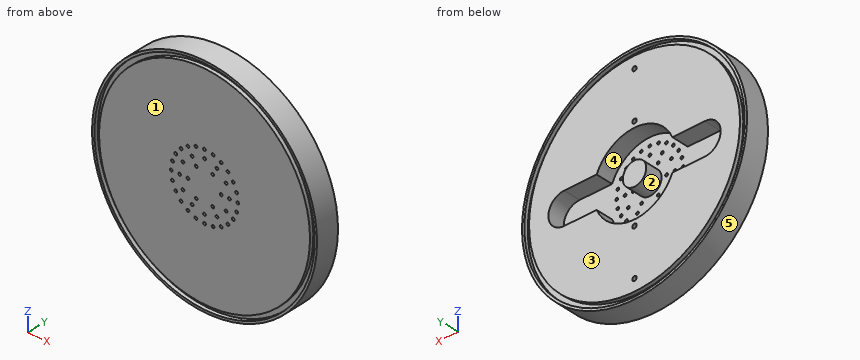
```python
from build123d import *

# Parameters (mm, degrees)
SKETCH1_R                       = 60.96
BILLET_DEPTH                    = 12.7
SKETCH4_R                       = 0.7493
FIRST_KEROSENE_OUTLET_DEPTH     = 88.140881336
SKETCH15_R                      = 59.69
SKETCH15_R_2                    = 57.15
CHAMBER_O_RING_DEPTH            = 2.032
TOP_START                       = -2.032
SKETCH16_R                      = 59.69
SKETCH16_R_2                    = 57.15
TOP_O_RING_DEPTH                = 2.032
PRIMARY_HOLES_COUNT             = 6
SECOND_START                    = -12.7
SECOND_RING_OUTLINE_R           = 0.7493
SECOND_RING_DEPTH               = 12.7
THIRD_START                     = -12.7
THIRD_RING_OUTLINE_R            = 0.7493
THIRD_RING_DEPTH                = 12.7
KEROSENE_WELL_DEPTH             = 9.3218
SKETCH17_R                      = 6.35
BOSS_EXTRUDE1_DEPTH             = 2.54
BOSS_EXTRUDE1_DIRECTION_2_REACH = 89.141
SKETCH19_R                      = 6.35
LOX_TOWER_DEPTH                 = 2.54
SKETCH20_R                      = 1.190625
DOWELS_DEPTH                    = 3.175


# Read off the part's stored shape, not the designer's step: Second ring, Third Ring
with BuildPart() as part:
    # Sketch1 → Billet (new body)
    with BuildSketch(Plane(origin=(0, 0, 0), x_dir=(1, 0, 0), z_dir=(0, 1, 0))):
        with Locations(Location((0, 0, 0), (0, 0, 270))):
            Circle(SKETCH1_R)
    extrude(amount=-BILLET_DEPTH)

    # Sketch4 → First Kerosene Outlet (cut, symmetric)
    with BuildSketch(Plane(origin=(0, -12.7, 0), x_dir=(1, 0, 0), z_dir=(0, 1, 0))):
        with Locations(Location((8.9916, 0, 0), (0, 0, 270))):
            Circle(SKETCH4_R)
        with Locations(Location((13.4874, 0, 0), (0, 0, 270))):
            Circle(SKETCH4_R)
        with Locations(Location((17.9832, 0, 0), (0, 0, 270))):
            Circle(SKETCH4_R)
    first_kerosene_outlet = extrude(amount=FIRST_KEROSENE_OUTLET_DEPTH, both=True, mode=Mode.SUBTRACT)

    # Sketch15 → Chamber O Ring (cut)
    with BuildSketch(Plane(origin=(0, -12.7, 0), x_dir=(1, 0, 0), z_dir=(0, 1, 0))):
        with Locations(Location((0, 0, 0), (0, 0, 270))):
            Circle(SKETCH15_R)
        with Locations(Location((0, 0, 0), (0, 0, 270))):
            Circle(SKETCH15_R_2, mode=Mode.SUBTRACT)
    extrude(amount=CHAMBER_O_RING_DEPTH, mode=Mode.SUBTRACT)

    # Sketch16 → Top O ring (cut)
    with BuildSketch(Plane(origin=(0, 0, 0), x_dir=(1, 0, 0), z_dir=(0, 1, 0)).offset(TOP_START)):
        with Locations(Location((0, 0, 0), (0, 0, 270))):
            Circle(SKETCH16_R)
        with Locations(Location((0, 0, 0), (0, 0, 270))):
            Circle(SKETCH16_R_2, mode=Mode.SUBTRACT)
    extrude(amount=TOP_O_RING_DEPTH, mode=Mode.SUBTRACT)

    # Primary Holes: First Kerosene Outlet ×6 about axis
    primary_holes_axis = Axis((0, 0, 0), (0, 1, 0))
    for i in range(1, PRIMARY_HOLES_COUNT):
        add(first_kerosene_outlet.rotate(primary_holes_axis, i * 360 / PRIMARY_HOLES_COUNT), mode=Mode.SUBTRACT)

    # Second ring outline → Second ring (cut)
    with BuildSketch(Plane(origin=(0, 0, 0), x_dir=(1, 0, 0), z_dir=(0, 1, 0)).offset(SECOND_START)):
        with Locations((11.680431031, 6.7437)):
            Circle(SECOND_RING_OUTLINE_R)
        with Locations((0, 13.4874)):
            Circle(SECOND_RING_OUTLINE_R)
        with Locations((-11.680431031, 6.7437)):
            Circle(SECOND_RING_OUTLINE_R)
        with Locations((-11.680431031, -6.7437)):
            Circle(SECOND_RING_OUTLINE_R)
        with Locations((0, -13.4874)):
            Circle(SECOND_RING_OUTLINE_R)
        with Locations((11.680431031, -6.7437)):
            Circle(SECOND_RING_OUTLINE_R)
    extrude(amount=SECOND_RING_DEPTH, mode=Mode.SUBTRACT)

    # Third Ring outline → Third Ring (cut)
    with BuildSketch(Plane(origin=(0, 0, 0), x_dir=(1, 0, 0), z_dir=(0, 1, 0)).offset(THIRD_START)):
        with Locations((17.370437319, 4.654394652)):
            Circle(THIRD_RING_OUTLINE_R)
        with Locations((15.573908041, 8.9916)):
            Circle(THIRD_RING_OUTLINE_R)
        with Locations((12.716042667, 12.716042667)):
            Circle(THIRD_RING_OUTLINE_R)
        with Locations((4.654394652, 17.370437319)):
            Circle(THIRD_RING_OUTLINE_R)
        with Locations((0, 17.9832)):
            Circle(THIRD_RING_OUTLINE_R)
        with Locations((-4.654394652, 17.370437319)):
            Circle(THIRD_RING_OUTLINE_R)
        with Locations((-12.716042667, 12.716042667)):
            Circle(THIRD_RING_OUTLINE_R)
        with Locations((-15.573908041, 8.9916)):
            Circle(THIRD_RING_OUTLINE_R)
        with Locations((-17.370437319, 4.654394652)):
            Circle(THIRD_RING_OUTLINE_R)
        with Locations((-17.370437319, -4.654394652)):
            Circle(THIRD_RING_OUTLINE_R)
        with Locations((-15.573908041, -8.9916)):
            Circle(THIRD_RING_OUTLINE_R)
        with Locations((-12.716042667, -12.716042667)):
            Circle(THIRD_RING_OUTLINE_R)
        with Locations((-4.654394652, -17.370437319)):
            Circle(THIRD_RING_OUTLINE_R)
        with Locations((0, -17.9832)):
            Circle(THIRD_RING_OUTLINE_R)
        with Locations((4.654394652, -17.370437319)):
            Circle(THIRD_RING_OUTLINE_R)
        with Locations((12.716042667, -12.716042667)):
            Circle(THIRD_RING_OUTLINE_R)
        with Locations((15.573908041, -8.9916)):
            Circle(THIRD_RING_OUTLINE_R)
        with Locations((17.370437319, -4.654394652)):
            Circle(THIRD_RING_OUTLINE_R)
    extrude(amount=THIRD_RING_DEPTH, mode=Mode.SUBTRACT)

    # Sketch18 → Kerosene Well (cut)
    with BuildSketch(Plane(origin=(0, 0, 0), x_dir=(1, 0, 0), z_dir=(0, 1, 0))):
        with BuildLine():
            Line((-38.1, 8.57504), (-20.504129194, 8.57504))
            ThreePointArc((-20.504129194, 8.57504), (0, 22.225), (20.504129194, 8.57504))
            Line((20.504129194, 8.57504), (38.1, 8.57504))
            ThreePointArc((38.1, 8.57504), (46.67504, 0), (38.1, -8.57504))
            Line((38.1, -8.57504), (20.504129194, -8.57504))
            ThreePointArc((20.504129194, -8.57504), (0, -22.225), (-20.504129194, -8.57504))
            Line((-20.504129194, -8.57504), (-38.1, -8.57504))
            ThreePointArc((-38.1, -8.57504), (-46.67504, 0), (-38.1, 8.57504))
        make_face()
    extrude(amount=-KEROSENE_WELL_DEPTH, mode=Mode.SUBTRACT)

    # Sketch17 → Boss-Extrude1 (add)
    with BuildSketch(Plane(origin=(0, 0, 0), x_dir=(1, 0, 0), z_dir=(0, 1, 0))):
        with Locations(Location((0, 0, 0), (0, 0, 270))):
            Circle(SKETCH17_R)
    extrude(amount=BOSS_EXTRUDE1_DEPTH)

    # Sketch17 → Boss-Extrude1 direction 2 (add, up to next)
    with BuildSketch(Plane(origin=(0, 0, 0), x_dir=(1, 0, 0), z_dir=(0, 1, 0)), mode=Mode.PRIVATE) as boss_extrude1_direction_2_sk1:
        with Locations(Location((0, 0, 0), (0, 0, 270))):
            Circle(SKETCH17_R)
    boss_extrude1_direction_2_tool1 = extrude(boss_extrude1_direction_2_sk1.sketch, amount=-BOSS_EXTRUDE1_DIRECTION_2_REACH, mode=Mode.PRIVATE) - part.part
    add(boss_extrude1_direction_2_tool1.solids().sort_by_distance((0, 0, 0))[0])

    # Sketch19 → Lox Tower (cut)
    with BuildSketch(Plane(origin=(0, 2.54, 0), x_dir=(1, 0, 0), z_dir=(0, 1, 0))):
        with Locations(Location((0, 0, 0), (0, 0, 270))):
            Circle(SKETCH19_R)
    extrude(amount=-LOX_TOWER_DEPTH, mode=Mode.SUBTRACT)

    # Sketch20 → Dowels (cut)
    with BuildSketch(Plane(origin=(0, 0, 0), x_dir=(1, 0, 0), z_dir=(0, 1, 0))):
        with Locations(Location((0, 25.4, 0), (0, 0, 270))):
            Circle(SKETCH20_R)
        with Locations(Location((0, -25.4, 0), (0, 0, 90))):
            Circle(SKETCH20_R)
        with Locations(Location((0, 50.8, 0), (0, 0, 270))):
            Circle(SKETCH20_R)
        with Locations(Location((0, -50.8, 0), (0, 0, 90))):
            Circle(SKETCH20_R)
    extrude(amount=-DOWELS_DEPTH, mode=Mode.SUBTRACT)


solid = part.part
```
Can you work these out from the model? Positions are in its coordinate system, mm. Face numbers are marked on the shaded views. A direction names the side the tool comes from. Coordinates: 2 decimals unless noted, no trailing zeros. Loops run counter-clockwise (first coordinate to the right, second up) from the corner with the lowest first, then second, coordinate; pieces in that order, holes last.
1) For pin 1 (1.2 mm diameter, centred on x = 6.74, z = 11.68, fed in from -Y); pin 2 (4 mm diameter, centred on x = 43, y = -7, fed in from +Z); pin 3 (4 mm diameter, centred on y = -4, z = 17.5, fed in from +X); pin 4 (2.5 mm diameter, centred on x = 17.37, z = 4.65, fed in from +Y), each with a flat end and sliding along its axis, tell me the tip position at first contact or that it passes through.
2) Imagine slicing it at B-B on z = -36. List the corners of the cut face in (x, y) for me.
3) Imagine slicing it at A-A on y = -7.5. List the corners of the cut face in (x, z) for me (3 decimals), plus the area to 3 significant figures.
4) Thinking about a two-plate mould opening in X: for the marked faces 3, 4 and 5, which applies, pulls with the +X half, pulls with the -X half, needs draft (parallel to the pull), parting line crosses it, or undercut?
5) Which directions (+Z, -Z, +X, -X, +Y, -Y) give clear straight access to the entire face, cutting with the end or side of a thin tool? Please do the marked faces 1 and 2.
6) I need wall thicknesses on probe 1 along X at (y, z) = (-1.25, -4.5); probe 2 along X at (y, z) = (-10.75, 31); probe 3 along X at (y, z) = (-0.5, 15.5). Which ranges of each line are inside material? Lowest first, please.
7) Imagine slicing it at C-C on x = 26. List the corners of the cut face in (y, z) for me, plus the area to 3 significant figures.
Completed:
1. pin 1: passes through
1. pin 2: stops at z = 45.11
1. pin 3: stops at x = 58.96
1. pin 4: stops at y = -9.32
2. outline: (-49.19, -12.7) - (-47.61, -12.7) - (-47.61, -10.67) - (-44.39, -10.67) - (-44.39, -12.7) - (44.39, -12.7) - (44.39, -10.67) - (47.61, -10.67) - (47.61, -12.7) - (49.19, -12.7) - (49.19, 0) - (47.61, 0) - (47.61, -2.03) - (44.39, -2.03) - (44.39, 0) - (-44.39, 0) - (-44.39, -2.03) - (-47.61, -2.03) - (-47.61, 0) - (-49.19, 0) - close
3. outline: circle Ø121.92 at (0, 0); circle Ø12.7 at (0, 0); hole (-38.1, -8.575) - (-20.504, -8.575) arc R22.225 ccw to (20.504, -8.575) - (38.1, -8.575) arc R8.575 ccw to (38.1, 8.575) - (20.504, 8.575) arc R22.225 ccw to (-20.504, 8.575) - (-38.1, 8.575) arc R8.575 ccw to start
3. area: 9,450 mm2
4. face 3: needs draft
4. face 4: undercut
4. face 5: parting line crosses it
5. face 1: +Z, -Z, +X, -X, -Y
5. face 2: +Y
6. probe 1: x = -60.79 to -59.52, -56.97 to -45.4, -4.48 to 4.48, 45.4 to 56.97, 59.52 to 60.79
6. probe 2: x = -52.49 to -51.01, -48.01 to 48.01, 51.01 to 52.49
6. probe 3: x = -58.96 to -57.64, -55.01 to -15.93, 15.93 to 55.01, 57.64 to 58.96
7. outline: (-12.7, -55.14) - (0, -55.14) - (0, -53.73) - (-2.03, -53.73) - (-2.03, -50.89) - (0, -50.89) - (0, -8.58) - (-9.32, -8.58) - (-9.32, 8.58) - (0, 8.58) - (0, 50.89) - (-2.03, 50.89) - (-2.03, 53.73) - (0, 53.73) - (0, 55.14) - (-12.7, 55.14) - (-12.7, 53.73) - (-10.67, 53.73) - (-10.67, 50.89) - (-12.7, 50.89) - (-12.7, -50.89) - (-10.67, -50.89) - (-10.67, -53.73) - (-12.7, -53.73) - close
7. area: 1,220 mm2
